Build history of the part. All positions in model axes, mm. A direction names the side the tool comes from. Coordinates: 2 decimals unless noted, no trailing zeros. Loops run counter-clockwise (first coordinate to the right, second up) from the corner with the lowest first, then second, coordinate; pieces in that order, holes last.
(1) Slice it at D-D (x = 89). Give the cut face in (y, z), and give its area (3 significant figures).
(2) Slice it at A-A (z = -5). Give the cut face in (x, y).
(3) Two-plate mould, pull along X, no slides. Class faces 1 (the face through (89.129, 1.479, -135.744)), 2 (the face through (149.06, 1.479, -135.586)), 3 (the face through (6.352, 1.479, -6.474)): pulls with the +X half, pulls with the -X half, needs draft (parallel to the pull), parting line crosses it, or undercut.
(4) Wall check: L1, parallel to Z at x = 199, y = 1.5; L2, parallel to Z at x = 37, y = 1; L3, parallel to X at y = 0.4, z = -25.5. Give the ranges that are in metal, low to high.
(5) Slice it at C-C (z = -65). Give the cut face in (x, y), and give its area (3 significant figures).
(6) Flat gauge pins, fed straight in: P1, Ø0.9, axis at x = 191, y = 2, coming from the -Z side; P2, Ø5.5, axis at x = 99, z = -137.5, coming from the +Y side; P3, Ø1.6, axis at x = 119, z = -27.5, coming from the -Y side. Where does each tip first touch, or does it go through?
(7) Tool access for faces 4 (the face through (78, 3, -72)), 5 (the face through (50.23, 1.52, -35.07)): list every direction of +Z, -Z, +X, -X, +Y, -Y with a clear straight run to the whole face (end or side of a thin tool).
(8) Slice it at B-B (x = 38.5). Give the cut face in (y, z).
from build123d import *

# Parameters (mm, degrees)
SKETCH_1_R          = 2
SKETCH_1_R_2        = 3.05
SKETCH_1_R_3        = 1.3
SKETCH_1_R_4        = 32.4
SKETCH_1_R_5        = 1.65
EXTRUDE_1_DEPTH     = 3
CUT_EXTRUDE_1_DEPTH = 249.859900346
FILLET_1_R          = 3


with BuildPart() as part:
    # ｽｹｯﾁ1 → ﾎﾞｽ - 押し出し1 (new body)
    with BuildSketch(Plane(origin=(0, 0, 0), x_dir=(1, 0, 0), z_dir=(0, 1, 0))):
        with BuildLine():
            Line((0, 130), (0, 0))
            Line((0, 0), (204, 0))
            Line((204, 0), (204, 130))
            Line((204, 130), (155.716771079, 130))
            Line((155.716771079, 130), (142.213938048, 141.330222216))
            ThreePointArc((142.213938048, 141.330222216), (136.886908691, 142.031538935), (134, 137.5))
            Line((134, 137.5), (134, 127.5))
            ThreePointArc((134, 127.5), (119, 112.5), (104, 127.5))
            Line((104, 127.5), (104, 130))
            Line((104, 130), (104, 137.5))
            ThreePointArc((104, 137.5), (101.113091309, 142.031538935), (95.786061952, 141.330222216))
            Line((95.786061952, 141.330222216), (82.283228921, 130))
            Line((82.283228921, 130), (0, 130))
        make_face()
        with Locations(Location((5, 5, 0), (0, 0, 270))):
            Circle(SKETCH_1_R, mode=Mode.SUBTRACT)
        with Locations(Location((78.058517369, 24.058517369, 0), (0, 0, 270))):
            Circle(SKETCH_1_R_2, mode=Mode.SUBTRACT)
        with Locations(Location((119, 5, 0), (0, 0, 270))):
            Circle(SKETCH_1_R, mode=Mode.SUBTRACT)
        with Locations(Location((119, 27.5, 0), (0, 0, 270))):
            Circle(SKETCH_1_R_3, mode=Mode.SUBTRACT)
        with Locations(Location((199, 5, 0), (0, 0, 270))):
            Circle(SKETCH_1_R, mode=Mode.SUBTRACT)
        with Locations(Location((159.941482631, 24.058517369, 0), (0, 0, 270))):
            Circle(SKETCH_1_R_2, mode=Mode.SUBTRACT)
        with Locations(Location((119, 65, 0), (0, 0, 270))):
            Circle(SKETCH_1_R_4, mode=Mode.SUBTRACT)
        with Locations(Location((66.023144428, 93.168293767, 0), (0, 0, 270))):
            Circle(SKETCH_1_R, mode=Mode.SUBTRACT)
        with Locations(Location((5, 125, 0), (0, 0, 270))):
            Circle(SKETCH_1_R, mode=Mode.SUBTRACT)
        with Locations(Location((78.058517369, 105.941482631, 0), (0, 0, 270))):
            Circle(SKETCH_1_R_2, mode=Mode.SUBTRACT)
        with Locations(Location((99, 117.5, 0), (0, 0, 270))):
            Circle(SKETCH_1_R_5, mode=Mode.SUBTRACT)
        with Locations(Location((99, 137.5, 0), (0, 0, 270))):
            Circle(SKETCH_1_R_5, mode=Mode.SUBTRACT)
        with Locations(Location((171.976855572, 93.168293767, 0), (0, 0, 270))):
            Circle(SKETCH_1_R, mode=Mode.SUBTRACT)
        with Locations(Location((139, 117.5, 0), (0, 0, 270))):
            Circle(SKETCH_1_R_5, mode=Mode.SUBTRACT)
        with Locations(Location((159.941482631, 105.941482631, 0), (0, 0, 270))):
            Circle(SKETCH_1_R_2, mode=Mode.SUBTRACT)
        with Locations(Location((199, 125, 0), (0, 0, 270))):
            Circle(SKETCH_1_R, mode=Mode.SUBTRACT)
        with Locations(Location((139, 137.5, 0), (0, 0, 270))):
            Circle(SKETCH_1_R_5, mode=Mode.SUBTRACT)
    extrude(amount=EXTRUDE_1_DEPTH)

    # ｽｹｯﾁ2 → ｶｯﾄ - 押し出し1 (cut, through all)
    with BuildSketch(Plane(origin=(0, 3, 0), x_dir=(1, 0, 0), z_dir=(0, 1, 0))):
        with BuildLine():
            ThreePointArc((44.669656263, 75), (50.881747913, 96.383175949), (63.098300563, 115))
            Line((63.098300563, 115), (15, 115))
            Line((15, 115), (15, 75))
            Line((15, 75), (44.669656263, 75))
        make_face()
        with BuildLine():
            Line((15, 15), (63.098300563, 15))
            ThreePointArc((63.098300563, 15), (50.881747913, 33.616824051), (44.669656263, 55))
            Line((44.669656263, 55), (15, 55))
            Line((15, 55), (15, 15))
        make_face()
    extrude(amount=-CUT_EXTRUDE_1_DEPTH, mode=Mode.SUBTRACT)

    # ﾌｨﾚｯﾄ1
    fillet_1_edges = [part.edges().sort_by_distance(p)[0] for p in [
        (63.098300563, 1.5, -115),
        (44.669656263, 1.5, -75),
        (15, 1.5, -75),
        (15, 1.5, -115),
        (44.669656263, 1.5, -55),
        (63.098300563, 1.5, -15),
        (15, 1.5, -15),
        (15, 1.5, -55),
    ]]
    fillet(fillet_1_edges, radius=FILLET_1_R)


solid = part.part
Response values:
1. outline: (0, -135.64) - (3, -135.64) - (3, -77.24) - (0, -77.24) - close; (0, -52.76) - (3, -52.76) - (3, 0) - (0, 0) - close
1. area: 333 mm2
2. outline: (0, 0) - (3, 0) - (3, 3) - (0, 3) - close; (7, 0) - (117, 0) - (117, 3) - (7, 3) - close; (121, 0) - (197, 0) - (197, 3) - (121, 3) - close; (201, 0) - (204, 0) - (204, 3) - (201, 3) - close
3. face 1: pulls with the -X half
3. face 2: pulls with the +X half
3. face 3: undercut
4. L1: z = -130 to -127, -123 to -7, -3 to 0
4. L2: z = -130 to -115, -75 to -55, -15 to 0
4. L3: x = 0 to 15, 55.24 to 75.37, 80.75 to 157.25, 162.63 to 204
5. outline: (0, 0) - (86.6, 0) - (86.6, 3) - (0, 3) - close; (151.4, 0) - (204, 0) - (204, 3) - (151.4, 3) - close
5. area: 418 mm2
6. P1: stops at z = -130
6. P2: stops at y = 3
6. P3: passes through
7. face 4: +Z, -Z, +X, -X, +Y
7. face 5: +Y, -Y
8. outline: (0, -130) - (3, -130) - (3, -115) - (0, -115) - close; (0, -75) - (3, -75) - (3, -55) - (0, -55) - close; (0, -15) - (3, -15) - (3, 0) - (0, 0) - close
